Source: CAD feature listing. Evaluate the final solid. Frame: model axes, mm. Face numbers are marked on the shaded views. A direction names the side the tool comes from. Coordinates: 2 decimals unless noted, no trailing zeros. Order: outer loops, then holes, each group sorted by start corner. A loop starts at its lowest first (then second) coordinate and runs counter-clockwise, first axis right, second up. Notation, with made-up numbers: (12, 79.5) -> (19, 79.5) arc R13 cw to (19, 83.5) -> close; hole circle Ø1 at (-19.75, 6.25). An arc over 180 degrees is marked (long way). Write item = value, one per line. Start each with the question number.
Item 1: Section query D-D (x = 20). Output: boundary loops of the cut face in (y, z).
Item 2: Section query B-B (x = 1.5). Output: boundary loops of the cut face in (y, z), then the cut area to 3 significant figures.
Item 3: Ray query, line 1 along X through (y, z) = (1.4, 0); line 2 along Y through (x, z) = (20, 4.1); line 3 along Z through (x, y) = (0, 0.4). Return the intervals inside material, ascending. Write a range as [from, to].
Item 4: Section query C-C (z = 0). Output: boundary loops of the cut face in (x, y), then the cut area to 3 significant figures.
Item 5: Set-up query: the marked faces 5, 6 and 7. Return all of +Z, -Z, +X, -X, +Y, -Y with unobstructed straight access to the full face (end or side cutting, diameter ignored); none if empty.
Item 6: Section query A-A (y = 2.5). Output: boundary loops of the cut face in (x, z).
Item 7: Contact query for flat-ended pins moving along their axis: pin 1 (3 mm diameter, centred on x = 31.5, z = 0.5, fed in from +Y); pin 2 (7.5 mm diameter, centred on x = 14, z = 1.5, fed in from +Y). Output: stop coordinate, or through.
Item 8: Mould query, pull axis X, two halves, no side actions, for the marked faces 1, 2, 3 and 4. Classes: released by +X, released by -X, zero draft, split by the parting line, or undercut.
```python
from build123d import *

# Parameters (mm, degrees)
BOSS_EXTRUDE1_DEPTH = 2
SKETCH2_R           = 2.5
BOSS_EXTRUDE2_DEPTH = 5.5
SKETCH3_R           = 2.5
CUT_EXTRUDE1_DEPTH  = 2


with BuildPart() as part:
    # Sketch1 → Boss-Extrude1 (new body)
    with BuildSketch(Plane(origin=(0, 0, 0), x_dir=(1, 0, 0), z_dir=(0, 1, 0))):
        with BuildLine():
            Line((0, 7.5), (40, 7.5))
            ThreePointArc((40, 7.5), (47.5, 0), (40, -7.5))
            Line((40, -7.5), (0, -7.5))
            ThreePointArc((0, -7.5), (-7.5, 0), (0, 7.5))
        make_face()
    extrude(amount=BOSS_EXTRUDE1_DEPTH)

    # Sketch2 → Boss-Extrude2 (add)
    with BuildSketch(Plane.XY.offset(7.5)):
        with BuildLine():
            Line((15.918750874, 17.040738272), (11, 2))
            Line((11, 2), (20, 2))
            Line((20, 2), (29, 2))
            Line((29, 2), (24.081249126, 17.040738272))
            ThreePointArc((24.081249126, 17.040738272), (20, 20), (15.918750874, 17.040738272))
        make_face()
        with Locations((20, 15.706053276)):
            Circle(SKETCH2_R, mode=Mode.SUBTRACT)
    boss_extrude2 = extrude(amount=-BOSS_EXTRUDE2_DEPTH)

    # Mirror1: Boss-Extrude2 across plane
    add(boss_extrude2.mirror(Plane.XY))

    # Sketch3 → Cut-Extrude1 (cut)
    with BuildSketch(Plane(origin=(0, 2, 0), x_dir=(1, 0, 0), z_dir=(0, 1, 0))):
        Circle(SKETCH3_R)
        with Locations((40, 0)):
            Circle(SKETCH3_R)
    extrude(amount=-CUT_EXTRUDE1_DEPTH, mode=Mode.SUBTRACT)


solid = part.part
```
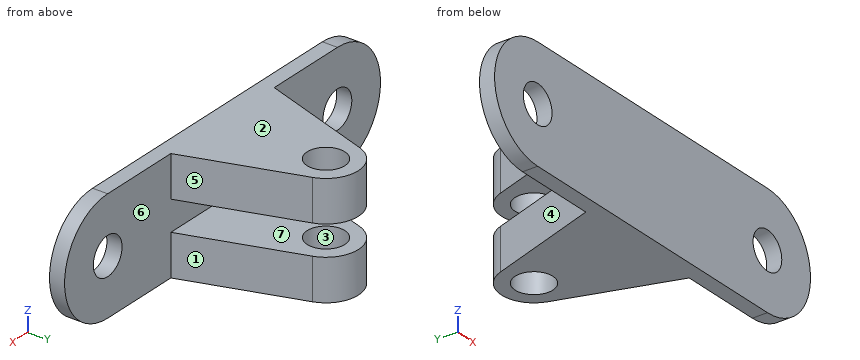
Computed:
q1.outline = (0, -7.5) -> (13.21, -7.5) -> (13.21, -2) -> (2, -2) -> (2, 2) -> (13.21, 2) -> (13.21, 7.5) -> (0, 7.5) -> close; (18.21, -7.5) -> (20, -7.5) -> (20, -2) -> (18.21, -2) -> close; (18.21, 2) -> (20, 2) -> (20, 7.5) -> (18.21, 7.5) -> close
q2.outline = (0, -7.5) -> (2, -7.5) -> (2, -2) -> (0, -2) -> close; (0, 2) -> (2, 2) -> (2, 7.5) -> (0, 7.5) -> close
q2.area = 22.0 mm^2
q3.line_1 = [-7.5, -2.5], [2.5, 37.5], [42.5, 47.5]
q3.line_2 = [0, 13.21], [18.21, 20]
q3.line_3 = [-7.5, -2.5], [2.5, 7.5]
q4.outline = (-7.5, 0) -> (-2.5, 0) -> (-2.5, 2) -> (-7.5, 2) -> close; (2.5, 0) -> (37.5, 0) -> (37.5, 2) -> (2.5, 2) -> close; (42.5, 0) -> (47.5, 0) -> (47.5, 2) -> (42.5, 2) -> close
q4.area = 90.0 mm^2
q5.face_5 = +Z, -Z, +X, +Y
q5.face_6 = +Y
q5.face_7 = +X, -X, +Y
q6.outline = (11.16, -7.5) -> (28.84, -7.5) -> (28.84, -2) -> (11.16, -2) -> close; (11.16, 2) -> (28.84, 2) -> (28.84, 7.5) -> (11.16, 7.5) -> close
q7.pin_1 = 2
q7.pin_2 = 19.34
q8.face_1 = released by +X
q8.face_2 = zero draft
q8.face_3 = undercut
q8.face_4 = released by -X
